The figure shows three views and two pictorial views of one solid part (mm, origin at its lowest corner). Answer the questions. Give positions to 0.01 mm unless a question says otherwise; leave off trailing zeros. Write each loop counter-clockwise with the first axis right and the second up, starting at its lowest first coordinate (ties: lowest second). Pieces come first, ordered by that corner, then holes. Notation, with made-up numbers: (-29, -31) - (15, -31) arc R9 ccw to (15, -19) - close; hole circle Ø10 at (41.5, 21.5). An arc over 180 degrees is marked (long way). Answer as CSV lines item,"result". Start each with the question number.
(1) Find section B-B (x = 16.5). Write down the section's boundary in (y, z) (1 decimal).
(2) Each of these flat-tipped pins is pushed along its axis until it touches: pin 1 Ø2 at (x, y) = (25.5, 14) entering from -Z; pin 2 Ø2 at (x, y) = (27, 75) entering from +Z; pin 3 Ø5 at (x, y) = (6, 32.5) entering from -Z. Where does it stop, or does it pass through?
(3) Straight lines are drawn through the part: probe 1 along Z at (x, y) = (35.5, 57.5); probe 2 along Z at (x, y) = (12, 24). For each, find the intervals that lie inside material, in ascending order.
(4) Find section A-A (y = 72.5). Write down the section's boundary in (x, z).
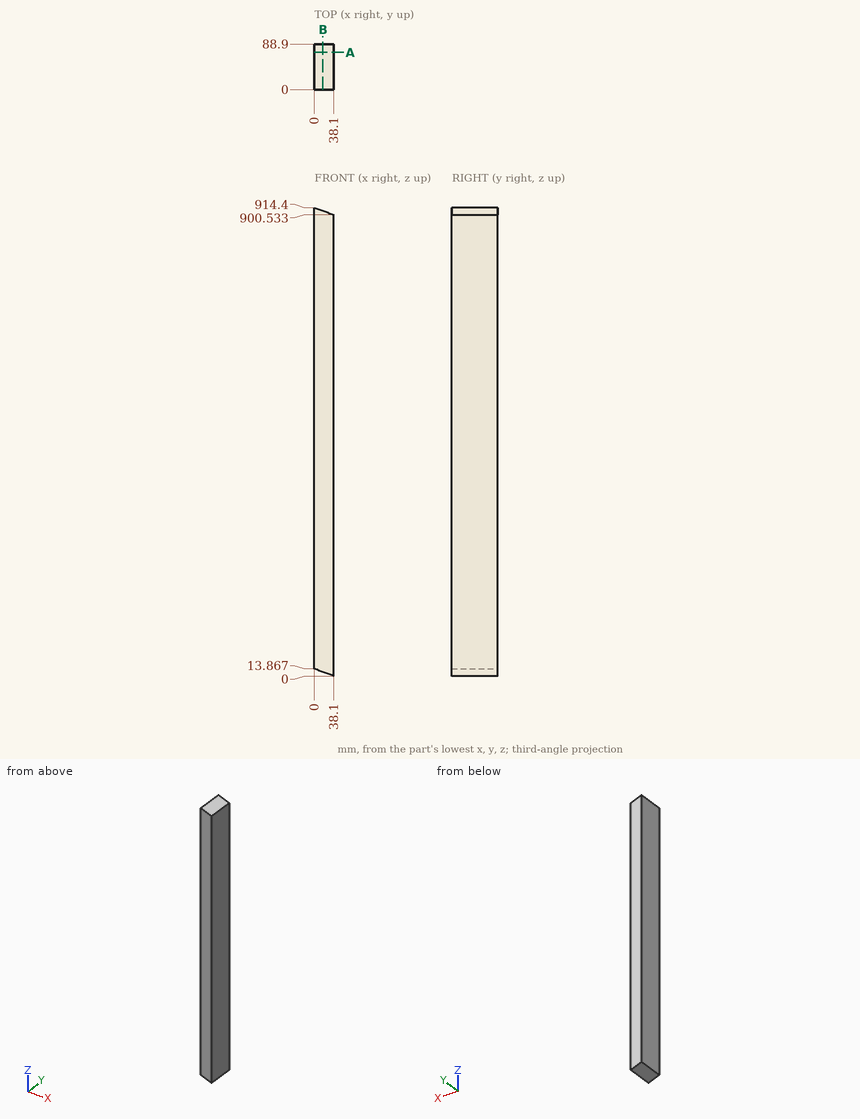
Result set:
1,outline,"(0, 7.9) - (88.9, 7.9) - (88.9, 908.4) - (0, 908.4) - close"
2,pin 1,"z = 4.22"
2,pin 2,"z = 904.94"
2,pin 3,"z = 10.77"
3,probe 1,"0.95 to 901.48"
3,probe 2,"9.5 to 910.03"
4,outline,"(0, 13.87) - (38.1, 0) - (38.1, 900.53) - (0, 914.4) - close"
